Work out the finished part from the listing and answer in its coordinate system (mm). A direction names the side the tool comes from. Give positions to 0.01 mm unless a question says otherwise; leave off trailing zeros. Loops run counter-clockwise (first coordinate to the right, second up) from the corner with the lowest first, then second, coordinate; pieces in that order, holes last. Notation, with made-up numbers: M 2.25,52.25 L 18.25,52.25 A5 cw 18.25,60.25 Z; hole C 19,10.5 d8. An arc over 180 degrees is marked long. Write item = value, one per line. Start each with the question number.
1. For faces 4 (the face through (15.5, 0.07, 2.46)), 5 (the face through (11.032, 10.873, 97.605)), 6 (the face through (-10.613, -9.879, 97.605)), 7 (the face through (7, 13, 90)), determine the directions among +Z, -Z, +X, -X, +Y, -Y from which every point of the face is accessible in a straight line to the end or side of a thin tool.
2. Flat-ended cylindrical pins translate along their axes: pin 1 Ø4 at (x, y) = (-7.5, -2.5) entering from -Z; pin 2 Ø2.5 at (x, y) = (0, -14) entering from -Z; pin 3 Ø1.5 at (y, z) = (-11, 24) entering from +X. Find the tip coordinate at first contact, or state that the pin passes through.
3. Section C-C on z = -8 is taken. Determine the outline of the cut face in (x, y), plus the area to 3 significant figures.
4. The mould has two halves that part along X. Classify faces 1 (the face through (0, 0, -20)), 2 (the face through (0.325, 12.536, 2.465)), 3 (the face through (12.932, -5.362, 46.905)): released by +X, released by -X, zero draft, split by the parting line, or undercut.
5. Section D-D on z = 49.5 is taken. Determine the outline of the cut face in (x, y).
6. Section A-A on y = 0 is taken. Determine the outline of the cut face in (x, z).
7. Consider L1, parallel to Y at x = 0, z = 3.7; L2, parallel to Z at x = -3.5, y = 0; L3, parallel to Z at x = 13, y = -9. Determine where each line is inside the solid, lowest interval first. Write a range as [from, to].
```python
from build123d import *

# Parameters (mm, degrees)
SKETCH1_R           = 18
BOSS_EXTRUDE1_DEPTH = 5
SKETCH2_R           = 14
BOSS_EXTRUDE2_DEPTH = 100
BOSS_EXTRUDE3_DEPTH = 15
SKETCH4_R           = 1.5
CUT_EXTRUDE1_DEPTH  = 5
SKETCH5_R           = 3
BOSS_EXTRUDE4_DEPTH = 20


with BuildPart() as part:
    # Sketch1 → Boss-Extrude1 (new body)
    with BuildSketch(Plane.XY):
        Circle(SKETCH1_R)
    extrude(amount=BOSS_EXTRUDE1_DEPTH)

    # Sketch2 → Boss-Extrude2 (add)
    with BuildSketch(Plane.XY.offset(5)):
        Circle(SKETCH2_R)
    extrude(amount=BOSS_EXTRUDE2_DEPTH)

    # Sketch3 → Boss-Extrude3 (add)
    with BuildSketch(Plane.XY.offset(105)):
        with BuildLine():
            Line((16.609319779, 5.29561128), (5.29561128, 16.609319779))
            Line((5.29561128, 16.609319779), (2.894461439, 14.208169938))
            ThreePointArc((2.894461439, 14.208169938), (-10.253048327, -10.253048327), (14.208169938, 2.894461439))
            Line((14.208169938, 2.894461439), (16.609319779, 5.29561128))
        make_face()
    extrude(amount=-BOSS_EXTRUDE3_DEPTH)

    # Sketch4 → Cut-Extrude1 (cut)
    with BuildSketch(Plane(origin=(0, 0, 0), x_dir=(-1, 0, 0), z_dir=(0, 0, -1))):
        with Locations((0, 14)):
            Circle(SKETCH4_R)
        with Locations((14, 0)):
            Circle(SKETCH4_R)
        with Locations((0, -14)):
            Circle(SKETCH4_R)
        with Locations((-14, 0)):
            Circle(SKETCH4_R)
    extrude(amount=-CUT_EXTRUDE1_DEPTH, mode=Mode.SUBTRACT)

    # Sketch5 → Boss-Extrude4 (add)
    with BuildSketch(Plane(origin=(0, 0, 0), x_dir=(-1, 0, 0), z_dir=(0, 0, -1))):
        with Locations(Location((0, 0, 0), (0, 0, 180))):
            Circle(SKETCH5_R)
    extrude(amount=BOSS_EXTRUDE4_DEPTH)


solid = part.part
```
Verdict:
q1.face_4 = -Z
q1.face_5 = +Z, +X, +Y
q1.face_6 = +Z
q1.face_7 = none
q2.pin_1 = 0
q2.pin_2 = 5
q2.pin_3 = 9.54
q3.outline = C 0,0 d6
q3.area = 28.3 mm2
q4.face_1 = zero draft
q4.face_2 = undercut
q4.face_3 = split by the parting line
q5.outline = C 0,0 d28
q6.outline = M -18,0 L -15.5,0 L -15.5,5 L -18,5 Z; M -14.5,90 L -14,90 L -14,5 L -12.5,5 L -12.5,0 L -3,0 L -3,-20 L 3,-20 L 3,0 L 12.5,0 L 12.5,5 L 14,5 L 14,90 L 14.5,90 L 14.5,105 L -14.5,105 Z; M 15.5,0 L 18,0 L 18,5 L 15.5,5 Z
q7.L1 = [-18, -15.5], [-12.5, 12.5], [15.5, 18]
q7.L2 = [0, 105]
q7.L3 = [0, 5]
